Source: CAD feature listing. Evaluate the final solid. Frame: model axes, mm. A direction names the side the tool comes from. Round coordinates to 2 decimals unless told otherwise and drop trailing zeros. Order: outer loops, then holes, each group sorted by start corner. A loop starts at its lowest first (then second) coordinate and runs counter-clockwise, first axis right, second up. Notation, with made-up numbers: M 16,-6.75 L 20,-6.75 A20 cw 20,12.25 Z; hole C 74,-10.5 d3. An arc over 180 degrees is marked long. Use one line per item in the form item = value. Start each with the question number.
Q1. Reachability of faces 4 (the conical face through (0.44, 1.35, 24.84)), 5 (the cylindrical face through (-8.6, 0, 5.1)), 6 (the conical face through (-0.12, 1.64, -10.14)) from +Z, -Z, +X, -X, +Y, -Y: full face, straight path, thin tool, end or side. Return the list, or none.
Q2. Material intervals for probe 1 along X at (y, z) = (-0.65, -12); probe 2 along X at (y, z) = (1.75, -10.75); probe 3 along X at (y, z) = (1.85, 21.5), sorted ascending.
Q3. Pull-direction query (Z, two-part tool) for faces 1 (the conical face through (15.404, 1.349, -9.737)), 2 (the cylindrical face through (0, 0, -18)), 3 (the flat face through (-6, 2, -10)); classes: pulls with the +Z half, pulls with the -Z half, needs draft (parallel to the pull), parting line crosses it, or undercut.
Q4. Section A-A (x = 0). Return the cut outline in (y, z), plus the area to 3 significant figures.
Q5. Contact query for flat-ended pins moving along their axis: pin 1 (5 mm diameter, centred on x = -18.62, z = -10.75, fed in from -Y); pin 2 (1 mm diameter, centred on x = 6.5, y = 1, fed in from -Z); pin 3 (0.7 mm diameter, centred on y = -1, z = 10.5, fed in from -X); pin 4 (1.5 mm diameter, centred on y = -1, z = 12.5, fed in from -X). Output: stop coordinate, or through.
Q6. Section B-B (y = -0.6). Return the cut outline in (x, z), plus the area to 3 significant figures.
from build123d import *

# Parameters (mm, degrees)
F0_R           = 10
F1_DEPTH       = 2
F1_DEPTH_BACK  = 2
F2_SIZE        = 0.5
F4_D           = 6.4
F4_CSINK_D     = 13.44
F4_CSINK_ANGLE = 90
F6_DEPTH       = 4.001


# Not quite as in the source:
# - a feature names something its author has since deleted; it is built from what else it names


with BuildPart() as f1:
    # F0 (on Front) → F1 (new body, two sides)
    with BuildSketch(Plane.XZ) as f1_sk:
        with BuildLine():
            ThreePointArc((10.7222839925, 14.457960644), (8.271877925, 17.429551948), (7.4940694571, 21.2018004501))
            ThreePointArc((7.4940694571, 21.2018004501), (0, 29), (-7.4940694571, 21.2018004501))
            ThreePointArc((-7.4940694571, 21.2018004501), (-8.271877925, 17.429551948), (-10.7222839925, 14.457960644))
            ThreePointArc((-10.7222839925, 14.457960644), (-15.5884572681, 9), (-17.8821032009, 2.0567900021))
            ThreePointArc((-17.8821032009, 2.0567900021), (-19.2303737261, -1.551119554), (-22.1083325243, -4.1108456974))
            ThreePointArc((-22.1083325243, -4.1108456974), (-25.1147367097, -14.5), (-14.6142630672, -17.0909547527))
            ThreePointArc((-14.6142630672, -17.0909547527), (-10.9584958011, -15.8784323941), (-7.1598192084, -16.5147506461))
            ThreePointArc((-7.1598192084, -16.5147506461), (0, -18), (7.1598192084, -16.5147506461))
            ThreePointArc((7.1598192084, -16.5147506461), (10.9584958011, -15.8784323941), (14.6142630672, -17.0909547527))
            ThreePointArc((14.6142630672, -17.0909547527), (25.1147367097, -14.5), (22.1083325243, -4.1108456974))
            ThreePointArc((22.1083325243, -4.1108456974), (19.2303737261, -1.551119554), (17.8821032009, 2.0567900021))
            ThreePointArc((17.8821032009, 2.0567900021), (15.5884572681, 9), (10.7222839925, 14.457960644))
        make_face()
        Circle(F0_R, mode=Mode.SUBTRACT)
    extrude(amount=F1_DEPTH)
    extrude(f1_sk.sketch, amount=-F1_DEPTH_BACK)

    # F2
    f2_edges = [f1.edges().sort_by_distance(p)[0] for p in [
        (0, -2, 29),
        (0, 2, 29),
        (-10, -2, 0),
        (-10, 2, 0),
    ]]
    chamfer(f2_edges, length=F2_SIZE)

    # F4 (through all)
    with Locations(Plane.XZ.offset(2)):
        with Locations((0, 21.5), (-18.6195461814, -10.75), (18.6195461814, -10.75)):
            CounterSinkHole(F4_D / 2, F4_CSINK_D / 2, counter_sink_angle=F4_CSINK_ANGLE)

    # F5 (on face) → F6 (cut, through all)
    with BuildSketch(Plane.XZ.offset(2)):
        with BuildLine():
            ThreePointArc((-2, 9.7979589711), (0, 10), (2, 9.7979589711))
            Line((2, 9.7979589711), (2, 12))
            ThreePointArc((2, 12), (0, 14), (-2, 12))
            Line((-2, 12), (-2, 9.7979589711))
        make_face()
        with BuildLine():
            Line((-9.3923048454, -7.7320508076), (-7.4852813742, -6.6310302931))
            ThreePointArc((-7.4852813742, -6.6310302931), (-8.6602540378, -5), (-9.4852813742, -3.166928678))
            Line((-9.4852813742, -3.166928678), (-11.3923048454, -4.2679491924))
            ThreePointArc((-11.3923048454, -4.2679491924), (-12.124355653, -7), (-9.3923048454, -7.7320508076))
        make_face()
        with BuildLine():
            Line((11.3923048454, -4.2679491924), (9.4852813742, -3.166928678))
            ThreePointArc((9.4852813742, -3.166928678), (8.6602540378, -5), (7.4852813742, -6.6310302931))
            Line((7.4852813742, -6.6310302931), (9.3923048454, -7.7320508076))
            ThreePointArc((9.3923048454, -7.7320508076), (12.124355653, -7), (11.3923048454, -4.2679491924))
        make_face()
    extrude(amount=-F6_DEPTH, mode=Mode.SUBTRACT)


solid = f1.part
Results list:
q1.face_4 = -Y
q1.face_5 = +Y, -Y
q1.face_6 = +Y
q2.probe_1 = -26.01 to -23.84, -13.4 to 13.4, 23.84 to 26.01
q2.probe_2 = -25.87 to -21.82, -15.42 to 15.42, 21.82 to 25.87
q2.probe_3 = -7.15 to -3.2, 3.2 to 7.15
q3.face_1 = undercut
q3.face_2 = pulls with the -Z half
q3.face_3 = needs draft
q4.outline = M -2,-17.5 L -1.5,-18 L 1.5,-18 L 2,-17.5 L 2,-10.5 L 1.5,-10 L -1.5,-10 L -2,-10.5 Z; M -2,14 L 2,14 L 2,18.3 L 1.52,18.3 L -2,14.78 Z; M -2,28.22 L 1.52,24.7 L 2,24.7 L 2,28.5 L 1.5,29 L -1.5,29 L -2,28.5 Z
q4.area = 53.3 mm2
q5.pin_1 = through
q5.pin_2 = -16.97
q5.pin_3 = -14.87
q5.pin_4 = -13.64
q6.outline = M -22.11,-4.11 A7.5 ccw long -14.61,-17.09 A8 cw -7.16,-16.51 A18 ccw 7.16,-16.51 A8 cw 14.61,-17.09 A7.5 ccw long 22.11,-4.11 A8 cw 17.88,2.06 A18 ccw 10.72,14.46 A8 cw 7.49,21.2 A7.5 ccw long -7.49,21.2 A8 cw -10.72,14.46 A18 ccw -17.88,2.06 A8 cw Z; hole C -18.62,-10.75 d10.64; hole M -11.39,-4.27 A2 ccw -9.39,-7.73 L -7.49,-6.63 A10 ccw 7.49,-6.63 L 9.39,-7.73 A2 ccw 11.39,-4.27 L 9.49,-3.17 A10 ccw 2,9.8 L 2,12 A2 ccw -2,12 L -2,9.8 A10 ccw -9.49,-3.17 Z; hole C 0,21.5 d10.64; hole C 18.62,-10.75 d10.64
q6.area = 857 mm2
